Check sheet for the modelled part. Datum: model origin and axes. Units: mm. Give positions to 0.01 mm unless a question says otherwise; leave off trailing zeros. Order: outer loops, then holes, each group sorted by start corner. A loop starts at its lowest first (then second) coordinate and runs counter-clockwise, first axis right, second up.
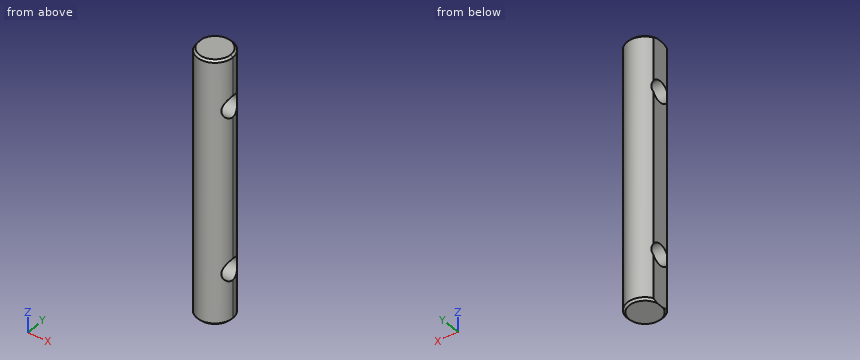
```python
from build123d import *

# Parameters (mm, degrees)
F1_DEPTH = 13
F2_SIZE  = 0.2
F4_D     = 2.1


with BuildPart() as f1:
    # F0 (on Top) → F1 (new body, symmetric)
    with BuildSketch(Plane.XY):
        with BuildLine():
            ThreePointArc((-1.5, -0.901388), (0.467707, -1.686342), (1.75, 0))
            ThreePointArc((1.75, 0), (0.467707, 1.686342), (-1.5, 0.901388))
            Line((-1.5, 0.901388), (-1.5, -0.901388))
        make_face()
    extrude(amount=F1_DEPTH, both=True)

    # F2
    f2_edges = [f1.edges().sort_by_distance(p)[0] for p in [
        (0.467707, 1.686342, 13),
        (0.467707, -1.686342, 13),
        (0.467707, 1.686342, -13),
        (0.467707, -1.686342, -13),
    ]]
    chamfer(f2_edges, length=F2_SIZE)

    # F4 (through all)
    with Locations(Plane(origin=(-1.5, 0, 0), x_dir=(0, -1, 0), z_dir=(-1, 0, 0))):
        with Locations((0, 8), (0, -8)):
            Hole(F4_D / 2)


solid = f1.part
```
(1) Go/stop test with a flat-tipped pin: P1, Ø1.5, axis at x = 1.5, y = -0.5, coming from the +Z side. Record where the tip stops, or that it passes through.
(2) Sectioned sample at C-C (x = 0.85). Count the separate pieces of the cut face and the enclosed holes in it, plus the area to 3 significant figures.
(3) Sectioned sample at A-A (z = 8). Enter the section's corners in (x, y), plus the area to 3 significant figures.
(4) Thickness scan on L1, parallel to Z at x = 0, y = 0; L2, parallel to Z at x = 1.5, y = 0.5; L3, parallel to Y at x = -0.6, z = -8. Record the ranges inside material, lowest first.
(5) Sectioned sample at B-B (z = -6.25). Enter the section's corners in (x, y), plus the area to 3 significant figures.
Values follow:
1. P1: stops at z = 13
2. separate pieces: 1
2. enclosed holes: 2
2. area: 72.5 mm2
3. outline: (-1.4, -1.05) arc R1.75 ccw to (1.4, -1.05) - close; (-1.4, 1.05) - (1.4, 1.05) arc R1.75 ccw to start
3. area: 2.74 mm2
4. L1: z = -13 to -9.05, -6.95 to 6.95, 9.05 to 13
4. L2: z = -12.97 to -8.92, -7.08 to 7.08, 8.92 to 12.97
4. L3: y = -1.64 to -1.05, 1.05 to 1.64
5. outline: (-1.5, -0.9) arc R1.75 ccw (long way) to (-1.5, 0.9) - close
5. area: 9.32 mm2
